Work out the finished part from the listing and answer in its coordinate system (mm). A direction names the side the tool comes from. Coordinates: 2 decimals unless noted, no trailing zeros. Order: outer loops, then holes, each group sorted by start corner. A loop starts at its lowest first (then second) coordinate and runs counter-clockwise, first axis right, second up. Notation, with made-up numbers: (-33, 13) -> (14, 13) arc R15 cw to (14, 38) -> close; hole circle Ø9 at (16.25, 35.5). An arc over 180 degrees is marked (long way). Use one line per item in the form item = value.
from build123d import *

# Parameters (mm, degrees)
SKETCH_1_W          = 70
SKETCH_1_H          = 50
EXTRUDE_1_DEPTH     = 3
EXTRUDE_2_DEPTH     = 70
SKETCH_3_R          = 1.6
EXTRUDE_3_DEPTH     = 3
EXTRUDE_4_REACH     = 139.875
SKETCH_4_W          = 70
SKETCH_4_H          = 5.267949192
FILLET_1_R          = 5
SKETCH_5_W          = 70
SKETCH_5_H          = 28.866025404
CUT_EXTRUDE_1_DEPTH = 138.47436204
SKETCH_6_W          = 70
SKETCH_6_H          = 3
CUT_EXTRUDE_2_DEPTH = 133.365261865
FILLET_2_R          = 5
SKETCH_7_R          = 1.6
CUT_EXTRUDE_3_DEPTH = 10
CUT_EXTRUDE_4_DEPTH = 10
CUT_EXTRUDE_5_DEPTH = 136.899592623
FILLET_4_R          = 10


with BuildPart() as part:
    # 草图1 → 凸台-拉伸1 (new body)
    with BuildSketch(Plane(origin=(0, 0, 0), x_dir=(1, 0, 0), z_dir=(0, 1, 0))):
        with Locations((35, 25)):
            Rectangle(SKETCH_1_W, SKETCH_1_H)
    extrude(amount=EXTRUDE_1_DEPTH)

    # 草图2 → 凸台-拉伸2 (add)
    with BuildSketch(Plane.ZY):
        Polygon((0, 15), (-6.062177826, 18.5), (-4.562177826, 21.098076211), (4, 16.154700538), (4, 15), (4, 0), (0, 0), align=None)
    extrude(amount=-EXTRUDE_2_DEPTH)

    # 草图3 → 凸台-拉伸3 (add)
    with BuildSketch(Plane(origin=(0, 13.848076211, 7.995190528), x_dir=(1, 0, 0), z_dir=(0, 0.86602540378444, 0.49999999999999784))):
        with BuildLine():
            Line((-48.265, 11.613248654), (-36.265, 11.613248654))
            Line((-36.265, 11.613248654), (106.265, 11.613248654))
            Line((106.265, 11.613248654), (118.265, 11.613248654))
            ThreePointArc((118.265, 11.613248654), (125.265, 4.613248654), (118.265, -2.386751346))
            Line((118.265, -2.386751346), (106.265, -2.386751346))
            Line((106.265, -2.386751346), (-36.265, -2.386751346))
            Line((-36.265, -2.386751346), (-48.265, -2.386751346))
            ThreePointArc((-48.265, -2.386751346), (-55.265, 4.613248654), (-48.265, 11.613248654))
        make_face()
        with Locations(Location((-36.265, 4.613248654, 0), (0, 0, 270))):
            Circle(SKETCH_3_R, mode=Mode.SUBTRACT)
        with Locations(Location((106.265, 4.613248654, 0), (0, 0, 270))):
            Circle(SKETCH_3_R, mode=Mode.SUBTRACT)
        with Locations(Location((-48.265, 4.613248654, 0), (0, 0, 270))):
            Circle(SKETCH_3_R, mode=Mode.SUBTRACT)
        with Locations(Location((118.265, 4.613248654, 0), (0, 0, 270))):
            Circle(SKETCH_3_R, mode=Mode.SUBTRACT)
    extrude(amount=-EXTRUDE_3_DEPTH)

    # 凸台-拉伸4: up to this face of the body (flat: up to its plane)
    extrude_4_end = Plane(part.part.faces().sort_by_distance((35, 6.345299462, 4))[0])
    # 草图4 → 凸台-拉伸4 (add, up to the picked face)
    with BuildSketch(Plane(origin=(0, 11.25, 6.495190528), x_dir=(1, 0, 0), z_dir=(0, -0.8660254037844396, -0.4999999999999982)), mode=Mode.PRIVATE) as extrude_4_sk1:
        with Locations((35, -0.24722325)):
            Rectangle(SKETCH_4_W, SKETCH_4_H)
    extrude_4_tool1 = split(extrude(extrude_4_sk1.sketch, amount=EXTRUDE_4_REACH, mode=Mode.PRIVATE), bisect_by=extrude_4_end, keep=Keep.BOTH, mode=Mode.PRIVATE)
    add(extrude_4_tool1.solids().sort_by(Axis((35, 11.373612, 6.281089), (0, -0.8660254037844396, -0.4999999999999982)))[0])

    # 圆角1
    fillet_1_edges = [part.edges().sort_by_distance(p)[0] for p in [
        (35, 3, 0),
    ]]
    fillet(fillet_1_edges, radius=FILLET_1_R)

    # 草图5 → 切除-拉伸1 (cut, through all)
    with BuildSketch(Plane(origin=(0, -1.193375673, 2.066987298), x_dir=(1, 0, 0), z_dir=(-1.4881366732147052e-15, -0.49999999999999784, 0.8660254037844398))):
        with Locations((35, -10.566987298)):
            Rectangle(SKETCH_5_W, SKETCH_5_H)
    extrude(amount=CUT_EXTRUDE_1_DEPTH, mode=Mode.SUBTRACT)

    # 草图6 → 切除-拉伸2 (cut, through all)
    with BuildSketch(Plane(origin=(0, 5.806624327, -10.057368355), x_dir=(-1, 0, 0), z_dir=(0, 0.49999999999999784, -0.8660254037844398))):
        with Locations((-35, 14.490381057)):
            Rectangle(SKETCH_6_W, SKETCH_6_H)
    extrude(amount=CUT_EXTRUDE_2_DEPTH, mode=Mode.SUBTRACT)

    # 圆角2
    fillet_2_edges = [part.edges().sort_by_distance(p)[0] for p in [
        (0, 1.5, -50),
        (70, 1.5, -50),
    ]]
    fillet(fillet_2_edges, radius=FILLET_2_R)

    # 草图7 → 切除-拉伸3 (cut)
    with BuildSketch(Plane(origin=(0, 3, 0), x_dir=(1, 0, 0), z_dir=(0, 1, 0))):
        with Locations(Location((10, 40, 0), (0, 0, 270))):
            Circle(SKETCH_7_R)
        with Locations(Location((60, 40, 0), (0, 0, 270))):
            Circle(SKETCH_7_R)
        with Locations(Location((35, 10, 0), (0, 0, 270))):
            Circle(SKETCH_7_R)
    extrude(amount=-CUT_EXTRUDE_3_DEPTH, mode=Mode.SUBTRACT)

    # 草图8 → 切除-拉伸4 (cut)
    with BuildSketch(Plane(origin=(0, 3, 0), x_dir=(1, 0, 0), z_dir=(0, 1, 0))):
        with BuildLine():
            ThreePointArc((31.364314075, 27.567539097), (33.020392023, 26.408578406), (35, 26))
            Line((35, 26), (35, 50))
            Line((35, 50), (7.167691896, 50))
            ThreePointArc((7.167691896, 50), (9.939143063, 49.427990232), (12.257652191, 47.805445265))
            Line((12.257652191, 47.805445265), (31.364314075, 27.567539097))
        make_face()
        with BuildLine():
            Line((35, 50), (35, 26))
            ThreePointArc((35, 26), (36.979607977, 26.408578406), (38.635685925, 27.567539097))
            Line((38.635685925, 27.567539097), (57.742347809, 47.805445265))
            ThreePointArc((57.742347809, 47.805445265), (60.060856937, 49.427990232), (62.832308104, 50))
            Line((62.832308104, 50), (35, 50))
        make_face()
    extrude(amount=-CUT_EXTRUDE_4_DEPTH, mode=Mode.SUBTRACT)

    # 草图9 → 切除-拉伸5 (cut, through all)
    with BuildSketch(Plane(origin=(0, 3, 0), x_dir=(1, 0, 0), z_dir=(0, 1, 0))):
        with BuildLine():
            Line((7, 29.511911518), (7, 12))
            ThreePointArc((7, 12), (8.025126266, 9.525126266), (10.5, 8.5))
            Line((10.5, 8.5), (24.5, 8.5))
            ThreePointArc((24.5, 8.5), (26.974873734, 9.525126266), (28, 12))
            Line((28, 12), (28, 19.543118511))
            ThreePointArc((28, 19.543118511), (27.752493698, 20.835900295), (27.044980148, 21.945841143))
            Line((27.044980148, 21.945841143), (16.795925867, 32.801709118))
            ThreePointArc((16.795925867, 32.801709118), (14.941700749, 33.830146274), (12.833963813, 33.599324324))
            ThreePointArc((12.833963813, 33.599324324), (11.611017181, 33.187906075), (10.333333333, 33.007941012))
            ThreePointArc((10.333333333, 33.007941012), (7.966885974, 31.927140976), (7, 29.511911518))
        make_face()
        with BuildLine():
            Line((42.955019852, 21.945841143), (53.204074133, 32.801709118))
            ThreePointArc((53.204074133, 32.801709118), (55.058299251, 33.830146274), (57.166036187, 33.599324324))
            ThreePointArc((57.166036187, 33.599324324), (58.388982819, 33.187906075), (59.666666667, 33.007941012))
            ThreePointArc((59.666666667, 33.007941012), (62.033114026, 31.927140976), (63, 29.511911518))
            Line((63, 29.511911518), (63, 12))
            ThreePointArc((63, 12), (61.974873734, 9.525126266), (59.5, 8.5))
            Line((59.5, 8.5), (45.5, 8.5))
            ThreePointArc((45.5, 8.5), (43.025126266, 9.525126266), (42, 12))
            Line((42, 12), (42, 19.543118511))
            ThreePointArc((42, 19.543118511), (42.247506302, 20.835900295), (42.955019852, 21.945841143))
        make_face()
    extrude(amount=-CUT_EXTRUDE_5_DEPTH, mode=Mode.SUBTRACT)

    # 圆角4
    fillet_4_edges = [part.edges().sort_by_distance(p)[0] for p in [
        (35, 0, 2.755983064),
    ]]
    fillet(fillet_4_edges, radius=FILLET_4_R)


solid = part.part
(1) Section C-C on x = -32 is taken. Write down the section's boundary in (y, z), plus the area to 3 significant figures.
Data:
outline = (10.06, 8.56) -> (17.06, -3.56) -> (19.65, -2.06) -> (12.65, 10.06) -> close
area = 42.0 mm²
(2) Straight lines are drawn through the part: line 1 along X through (y, z) = (1.2, -40); line 2 along X through (y, z) = (1.4, -10); line 3 along X through (y, z) = (2.5, -43.5). For each, find the intervals that lie inside material, in ascending order.
Data:
line_1 = 0 to 8.4, 11.6 to 19.63, 50.37 to 58.4, 61.6 to 70
line_2 = 0 to 7.63, 27.37 to 33.4, 36.6 to 42.63, 62.37 to 70
line_3 = 0 to 16.32, 53.68 to 70
(3) Each of these flat-tipped pins is pushed along its axis until it touches: P1, Ø2, axis at y = 2, z = -20.5, coming from the -X side; P2, Ø0.9, axis at x = 51.5, y = 1.5, coming from the -Z side; P3, Ø1.5, axis at x = 80, y = 10, coming from the +Z side; P4, Ø3, axis at x = 10, z = -40, coming from the -Y side. Where does it stop, or does it pass through?
Data:
P1 = 0
P2 = -41.67
P3 = 8.96
P4 = through
(4) The mould has two halves that part along Z. Classify faces 4 (the flat face through (35, 11, 0)), 5 (the flat face through (35, 3, -23)), 6 (the flat face through (21.99, 1.52, -27.3)): released by +Z, released by -Z, zero draft, split by the parting line, or undercut.
Data:
face_4 = released by -Z
face_5 = zero draft
face_6 = undercut
(5) Which of the six approach directions +Z, -Z, +X, -X, +Y, -Y give full straight-line access (tool end or side, diameter ignored) to faces 1 (the cylindrical face through (119.61, 14.44, 4.01)), 2 (the cylindrical face through (60, 1.5, -49.4)), 3 (the flat face through (48.01, 1.52, -27.3))?
Data:
face_1 = none
face_2 = -Z, +Y, -Y
face_3 = +Y, -Y
(6) Section A-A on x = 55.5 is taken. Write down the section's boundary in (y, z).
Data:
outline = (0, -45.43) -> (3, -45.43) -> (3, -33.89) -> (0, -33.89) -> close; (0, -8.5) -> (3, -8.5) -> (3, -5) arc R5 cw to (8, 0) -> (15, 0) -> (17.06, -3.56) -> (19.65, -2.06) -> (12.65, 10.06) -> (5, 5.64) arc R10 ccw to (0, -3.02) -> close
(7) Section B-B on z = -40 is taken. Write down the section's boundary in (x, y).
Data:
outline = (0, 0) -> (8.4, 0) -> (8.4, 3) -> (0, 3) -> close; (11.6, 0) -> (19.63, 0) -> (19.63, 3) -> (11.6, 3) -> close; (50.37, 0) -> (58.4, 0) -> (58.4, 3) -> (50.37, 3) -> close; (61.6, 0) -> (70, 0) -> (70, 3) -> (61.6, 3) -> close
